Geometry: final body of the model. Coordinates: model frame, mm. A direction names the side the tool comes from. Give positions to 0.01 mm unless a question says otherwise; leave off trailing zeros. Order: outer loops, then holes, each group sorted by start corner. A loop starts at its lowest first (then second) coordinate and runs counter-clockwise, first axis right, second up. Notation, with made-up numbers: (-20.75, 78) -> (-12.75, 78) arc R22 ccw to (-12.75, 93) -> close; hole circle Ø2 at (50, 57.25). An arc over 180 degrees is marked (long way). Answer in a Markdown table with one row per item. Add a question column.
Q1. Cut plane A-A on z = 19.05. Return the cut outline in (x, y).
Q2. Cut plane B-B on y = 0. Return the cut outline in (x, z), and give its area (3 significant figures).
Q3. Line query: line 1 along Y through (x, z) = (3, 19); line 2 along Y through (x, z) = (30, -19.5); line 3 along Y through (x, z) = (7, -37). Output: solid intervals per line, ascending. Write a range as from..to.
Q4. Cut plane C-C on x = 29. Return the cut outline in (y, z), and give its area (3 significant figures).
Q5. Pull-direction query (Z, two-part tool) for faces 1 (the face through (40.623, 0.22, 24.045)), 2 (the face through (43, 12, 44.45)), 3 (the face through (70.4, 19, 1)), 4 (the face through (43, 12, -44.45)); classes: +Z half, -Z half, draft (parallel to the pull), parting line (faces both ways), or undercut.
Q6. Set-up query: faces 5 (the face through (45, 26, 1)), 6 (the face through (5.07, 0.123, -16.253)), 7 (the face through (10, -2.2, -21.2)). Return all of +Z, -Z, +X, -X, +Y, -Y with unobstructed straight access to the full face (end or side cutting, diameter ignored); none if empty.
Q7. Contact query for flat-ended pins moving along their axis: P1, Ø1.5, axis at x = 16, z = 14.5, coming from the +Y side; P2, Ø6, axis at y = 25.5, z = -14, coming from the -X side; P3, Ø3, axis at y = 1, z = 20, coming from the +X side; P4, Ø3.5, axis at y = 0, z = -19.05, coming from the -X side. Output: stop coordinate, or through.
Q8. Cut plane D-D on z = 35.5. Return the cut outline in (x, y).
from build123d import *

# Parameters (mm, degrees)
BOSS_EXTRUDE1_DEPTH = 44.45
SKETCH2_R           = 2.8
CUT_EXTRUDE1_DEPTH  = 98.532571483
SKETCH3_R           = 5
CUT_EXTRUDE2_DEPTH  = 60.4


with BuildPart() as part:
    # Sketch1 → Boss-Extrude1 (new, symmetric)
    with BuildSketch(Plane.XY):
        Polygon((70.4, 50.8), (57.7, 50.8), (45, 38.1), (45, 12.7), (0, 12.7), (0, -12.7), (70.4, -12.7), align=None)
    extrude(amount=BOSS_EXTRUDE1_DEPTH, both=True)

    # Sketch2 → Cut-Extrude1 (cut, through all)
    with BuildSketch(Plane(origin=(70.4, 0, 0), x_dir=(0, 0, -1), z_dir=(1, 0, 0))):
        with Locations((-19.05, 0)):
            Circle(SKETCH2_R)
        with Locations((19.05, 0)):
            Circle(SKETCH2_R)
    extrude(amount=-CUT_EXTRUDE1_DEPTH, mode=Mode.SUBTRACT)

    # Sketch3 → Cut-Extrude2 (cut)
    with BuildSketch(Plane(origin=(70.4, 0, 0), x_dir=(0, 0, -1), z_dir=(1, 0, 0))):
        with Locations((-19.05, 0)):
            Circle(SKETCH3_R)
        with Locations((19.05, 0)):
            Circle(SKETCH3_R)
    extrude(amount=-CUT_EXTRUDE2_DEPTH, mode=Mode.SUBTRACT)


solid = part.part
Completed:
| question | item | result |
|---|---|---|
| 1 | outline | (0, -12.7) -> (70.4, -12.7) -> (70.4, -5) -> (10, -5) -> (10, -2.8) -> (0, -2.8) -> close; (0, 2.8) -> (10, 2.8) -> (10, 5) -> (70.4, 5) -> (70.4, 50.8) -> (57.7, 50.8) -> (45, 38.1) -> (45, 12.7) -> (0, 12.7) -> close |
| 2 | outline | (0, -44.45) -> (70.4, -44.45) -> (70.4, -24.05) -> (10, -24.05) -> (10, -21.85) -> (0, -21.85) -> close; (0, -16.25) -> (10, -16.25) -> (10, -14.05) -> (70.4, -14.05) -> (70.4, 14.05) -> (10, 14.05) -> (10, 16.25) -> (0, 16.25) -> close; (0, 21.85) -> (10, 21.85) -> (10, 24.05) -> (70.4, 24.05) -> (70.4, 44.45) -> (0, 44.45) -> close |
| 2 | area | 4,940 mm² |
| 3 | line 1 | y = -12.7..-2.8, 2.8..12.7 |
| 3 | line 2 | y = -12.7..-4.98, 4.98..12.7 |
| 3 | line 3 | y = -12.7..12.7 |
| 4 | outline | (-12.7, -44.45) -> (12.7, -44.45) -> (12.7, 44.45) -> (-12.7, 44.45) -> close; hole circle Ø10 at (0, -19.05); hole circle Ø10 at (0, 19.05) |
| 4 | area | 2,100 mm² |
| 5 | face 1 | undercut |
| 5 | face 2 | +Z half |
| 5 | face 3 | draft |
| 5 | face 4 | -Z half |
| 6 | face 5 | +Z, -Z, -X, +Y |
| 6 | face 6 | +X, -X |
| 6 | face 7 | +X |
| 7 | P1 | stops at y = 12.7 |
| 7 | P2 | stops at x = 45 |
| 7 | P3 | stops at x = 10 |
| 7 | P4 | passes through |
| 8 | outline | (0, -12.7) -> (70.4, -12.7) -> (70.4, 50.8) -> (57.7, 50.8) -> (45, 38.1) -> (45, 12.7) -> (0, 12.7) -> close |
